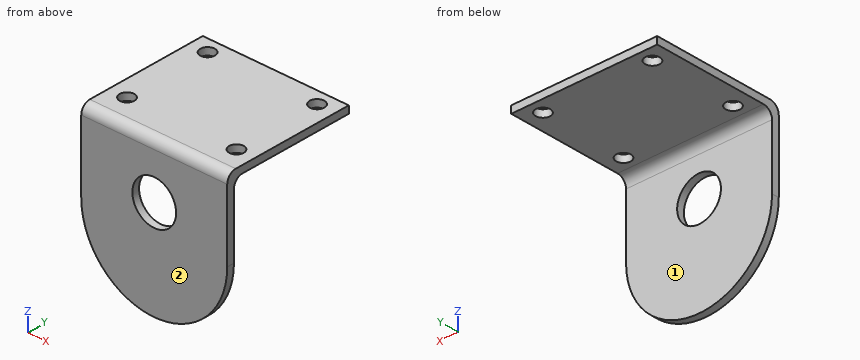
```python
from build123d import *

# Parameters (mm, degrees)
SKETCH1_W               = 40.005
SKETCH1_H               = 36.195
BOSS_EXTRUDE1_DEPTH     = 2
BOSS_EXTRUDE3_DEPTH     = 2
FILLET1_R               = 2.54
SKETCH4_R               = 2
CUT_EXTRUDE1_DEPTH      = 49.245409238
CUT_EXTRUDE2_DEPTH      = 58.534146654
CUT_EXTRUDE2_DEPTH_BACK = 58.534146654
SKETCH5_R               = 6


with BuildPart() as part:
    # Sketch1 → Boss-Extrude1 (new body)
    with BuildSketch(Plane.XY):
        Rectangle(SKETCH1_W, SKETCH1_H)
    extrude(amount=BOSS_EXTRUDE1_DEPTH)

    # Sketch3 → Boss-Extrude3 (add)
    with BuildSketch(Plane.XZ.offset(18.0975)):
        with BuildLine():
            Line((20.0025, 0), (-20.0025, 0))
            Line((-20.0025, 0), (-20.0025, -19.9975))
            ThreePointArc((-20.0025, -19.9975), (0, -40), (20.0025, -19.9975))
            Line((20.0025, -19.9975), (20.0025, 0))
        make_face()
    extrude(amount=-BOSS_EXTRUDE3_DEPTH)

    # Fillet1
    fillet1_edges = [part.edges().sort_by_distance(p)[0] for p in [
        (0, -16.0975, 0),
        (0, -18.0975, 2),
    ]]
    fillet(fillet1_edges, radius=FILLET1_R)

    # Sketch4 → Cut-Extrude1 (cut, through all)
    with BuildSketch(Plane(origin=(0, 0, 0), x_dir=(-1, 0, 0), z_dir=(0, 0, -1))):
        with Locations((-15.0025, 14.0975)):
            Circle(SKETCH4_R)
        with Locations((15.0025, 14.0975)):
            Circle(SKETCH4_R)
        with Locations((15.0025, -9.9025)):
            Circle(SKETCH4_R)
        with Locations((-15.0025, -9.9025)):
            Circle(SKETCH4_R)
    extrude(amount=-CUT_EXTRUDE1_DEPTH, mode=Mode.SUBTRACT)

    # Sketch5 → Cut-Extrude2 (cut, two sides: drawn at the far end of the back side and taken through both)
    with BuildSketch(Plane.XZ.offset(18.0975).offset(-CUT_EXTRUDE2_DEPTH_BACK)):
        with Locations(Location((0, -13, 0), (0, 0, 270))):
            Circle(SKETCH5_R)
    extrude(amount=CUT_EXTRUDE2_DEPTH + CUT_EXTRUDE2_DEPTH_BACK, mode=Mode.SUBTRACT)


solid = part.part
```
Part model, mm, in its own coordinate system. Face numbers are marked on the shaded views. A direction names the side the tool comes from. Give positions to 0.01 mm unless a question says otherwise; leave off trailing zeros. Write each loop counter-clockwise with the first axis right and the second up, starting at its lowest first coordinate (ties: lowest second). Pieces come first, ordered by that corner, then holes. Notation, with made-up numbers: (46.25, -7) -> (77.25, -7) arc R21 ccw to (77.25, 4) -> close; hole circle Ø1 at (76, 81). An arc over 180 degrees is marked (long way). Put each result on its own line as item: value. Start each with the question number.
Item 1: Cut at A-A (z = -13). List the corners of the cut face in (x, y).
Item 2: Cut at C-C (x = 14). List the corners of the cut face in (y, z), then the cut area to 3 significant figures.
Item 3: Which spindle directions (+Z, -Z, +X, -X, +Y, -Y) get a long thin tool onto all of the face, cutting with end or side? Do the marked faces 1 and 2. Say none if no direction does.
Item 4: Pin check, flat tip, straight feed: pin 1 Ø6.5 at (x, y) = (15, -9.9) entering from -Z. Stop position of the tip, or through.
Item 5: Cut at D-D (x = -11). List the corners of the cut face in (y, z), then the cut area to 3 significant figures.
Item 6: Wall check: L1, parallel to Z at x = -15, y = -2; L2, parallel to Y at x = 10, z = -19; L3, parallel to Z at x = 0, y = -16.7. Give the ranges that are in metal, low to high. Write a range as [from, to].
Item 7: Cut at B-B (x = -2.5). List the corners of the cut face in (y, z).
Answer list:
1. outline: (-20, -18.1) -> (-6, -18.1) -> (-6, -16.1) -> (-20, -16.1) -> close; (6, -18.1) -> (20, -18.1) -> (20, -16.1) -> (6, -16.1) -> close
2. outline: (-18.1, -34.28) -> (-16.1, -34.28) -> (-16.1, -2.54) arc R2.54 cw to (-13.56, 0) -> (-11.63, 0) -> (-11.63, 2) -> (-15.56, 2) arc R2.54 ccw to (-18.1, -0.54) -> close; (-8.17, 0) -> (12.37, 0) -> (12.37, 2) -> (-8.17, 2) -> close; (15.83, 0) -> (18.1, 0) -> (18.1, 2) -> (15.83, 2) -> close
2. area: 127 mm2
3. face 1: -Z, +X, -X, +Y
3. face 2: +Z, -Z, +X, -X, -Y
4. pin 1: stops at z = 0
5. outline: (-18.1, -36.7) -> (-16.1, -36.7) -> (-16.1, -2.54) arc R2.54 cw to (-13.56, 0) -> (18.1, 0) -> (18.1, 2) -> (-15.56, 2) arc R2.54 ccw to (-18.1, -0.54) -> close
5. area: 146 mm2
6. L1: z = [0, 2]
6. L2: y = [-18.1, -16.1]
6. L3: z = [-40, -19], [-7, 1.73]
7. outline: (-18.1, -39.84) -> (-16.1, -39.84) -> (-16.1, -18.45) -> (-18.1, -18.45) -> close; (-18.1, -7.55) -> (-16.1, -7.55) -> (-16.1, -2.54) arc R2.54 cw to (-13.56, 0) -> (18.1, 0) -> (18.1, 2) -> (-15.56, 2) arc R2.54 ccw to (-18.1, -0.54) -> close
